Check sheet for the modelled part. Datum: model origin and axes. Units: mm. A direction names the side the tool comes from. Round coordinates to 2 decimals unless told otherwise and drop trailing zeros. Write each loop counter-clockwise with the first axis right and the second up, starting at its lowest first coordinate (ties: lowest second). Pieces come first, ordered by that corner, then holes. Notation, with made-up numbers: (29, 36) -> (54, 36) arc R35 ccw to (54, 69) -> close; hole circle Ø3 at (87.5, 58.25). An arc over 180 degrees is marked (long way). One line per item, written item: value.
from build123d import *

# Parameters (mm, degrees)
F1_DEPTH = 20
F2_START = 1.5
F2_DEPTH = 17
F3_W     = 17
F3_H     = 17
F4_DEPTH = 30
F5_W     = 17
F5_H     = 17
F6_DEPTH = 30


with BuildPart() as f1:
    # F0 (on Top) → F1 (new body)
    with BuildSketch(Plane.XY):
        Polygon((8.5, -10), (10, -10), (10, 10), (-10, 10), (-10, 8.5), (-10, 0), (-10, -8.5), (-10, -10), (-8.5, -10), (0, -10), align=None)
    extrude(amount=F1_DEPTH)

    # F0 (on Top) → F2 (join)
    with BuildSketch(Plane.XY.offset(F2_START)):
        Polygon((-10, 0), (-10, 8.5), (-40, 8.5), (-40, -8.5), (-10, -8.5), align=None)
    extrude(amount=F2_DEPTH)

    # F3 (on face) → F4 (join)
    with BuildSketch(Plane.XY.offset(20)):
        Rectangle(F3_W, F3_H)
    extrude(amount=F4_DEPTH)

    # F5 (on face) → F6 (join)
    with BuildSketch(Plane(origin=(0, 0, 0), x_dir=(1, 0, 0), z_dir=(0, 0, -1))):
        Rectangle(F5_W, F5_H)
    extrude(amount=F6_DEPTH)


solid = f1.part
Item 1: Sectioned sample at B-B on y = 4.5. Enter the section's corners in (x, z).
Answer:
outline: (-40, 1.5) -> (-10, 1.5) -> (-10, 0) -> (-8.5, 0) -> (-8.5, -30) -> (8.5, -30) -> (8.5, 0) -> (10, 0) -> (10, 20) -> (8.5, 20) -> (8.5, 50) -> (-8.5, 50) -> (-8.5, 20) -> (-10, 20) -> (-10, 18.5) -> (-40, 18.5) -> close
Item 2: Sectioned sample at D-D on x = -35. Enter the section's corners in (y, z).
Answer:
outline: (-8.5, 1.5) -> (8.5, 1.5) -> (8.5, 18.5) -> (-8.5, 18.5) -> close
Item 3: Sectioned sample at C-C on z = -11. Enter the section's corners in (x, y).
Answer:
outline: (-8.5, -8.5) -> (8.5, -8.5) -> (8.5, 8.5) -> (-8.5, 8.5) -> close
Item 4: Tool access check on faces 1 (the flat face through (0, -8.5, 35)), 2 (the flat face through (0, 8.5, 35)), 3 (the flat face through (8.5, 0, 35)), 4 (the flat face through (-8.5, 0, 35)). Record the directions out of +Z, -Z, +X, -X, +Y, -Y that give a thin tool (end or side, any length) a straight path to the whole face; none if there is none.
Answer:
face 1: +Z, +X, -X, -Y
face 2: +Z, +X, -X, +Y
face 3: +Z, +X, +Y, -Y
face 4: +Z, -X, +Y, -Y
Item 5: Depth check by flat-ended pin: P1, Ø1, axis at y = 3.5, z = 39.5, coming from the +X side; P2, Ø5, axis at x = -2.5, z = 37.5, coming from the +Y side; P3, Ø4, axis at x = -19, y = 1, coming from the +Z side. Enter the tip coordinate at first touch or a pass-through.
Answer:
P1: stops at x = 8.5
P2: stops at y = 8.5
P3: stops at z = 18.5
Item 6: Sectioned sample at A-A on x = -1.5. Enter the section's corners in (y, z), and give its area (3 significant figures).
Answer:
outline: (-10, 0) -> (-8.5, 0) -> (-8.5, -30) -> (8.5, -30) -> (8.5, 0) -> (10, 0) -> (10, 20) -> (8.5, 20) -> (8.5, 50) -> (-8.5, 50) -> (-8.5, 20) -> (-10, 20) -> close
area: 1,420 mm^2
Item 7: Thickness scan on line 1 (X direction, y = -3.5, z = -16); line 2 (X direction, y = 9, z = 11.5); line 3 (Z direction, x = -35, y = 1). Record the ranges inside material, lowest first.
Answer:
line 1: x = -8.5 to 8.5
line 2: x = -10 to 10
line 3: z = 1.5 to 18.5
